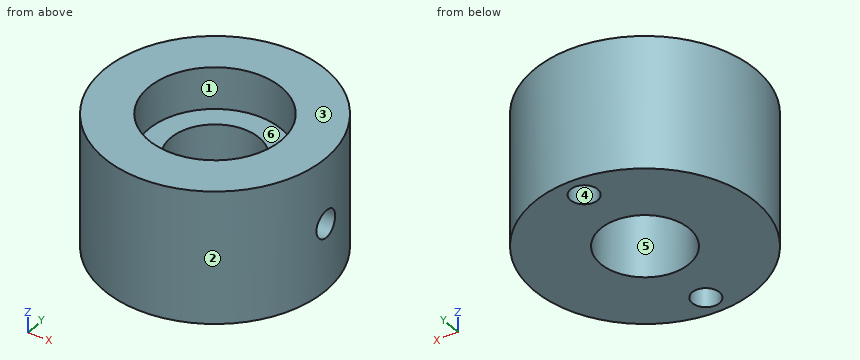
```python
from build123d import *

# Parameters (mm, degrees)
SKETCH1_R               = 15.875
SKETCH1_R_2             = 9.5
BOSS_EXTRUDE1_DEPTH     = 6
BOSS_EXTRUDE2_START     = -13.050000062
SKETCH1_3_R             = 15.875
SKETCH1_3_R_2           = 9.5
SKETCH1_3_R_3           = 6.35
BOSS_EXTRUDE2_DEPTH     = 13.050000062
SKETCH3_R               = 1.95
CUT_EXTRUDE1_DEPTH      = 10.16
CUT_EXTRUDE2_REACH      = 39.82
CUT_EXTRUDE2_END_RADIUS = 9.5


with BuildPart() as part:
    # Sketch1 → Boss-Extrude1 (new body)
    with BuildSketch(Plane.XY):
        Circle(SKETCH1_R)
        Circle(SKETCH1_R_2, mode=Mode.SUBTRACT)
    extrude(amount=BOSS_EXTRUDE1_DEPTH)

    # Sketch1<3> → Boss-Extrude2 (add)
    # profile 1 of 2: a face of its own
    with BuildSketch(Plane.XY.offset(BOSS_EXTRUDE2_START)):
        Circle(SKETCH1_3_R)
        Circle(SKETCH1_3_R_2, mode=Mode.SUBTRACT)
    # profile 2 of 2: a face of its own
    with BuildSketch(Plane.XY.offset(BOSS_EXTRUDE2_START)):
        Circle(SKETCH1_3_R_2)
        Circle(SKETCH1_3_R_3, mode=Mode.SUBTRACT)
    extrude(amount=BOSS_EXTRUDE2_DEPTH)

    # Sketch3 → Cut-Extrude1 (cut)
    with BuildSketch(Plane(origin=(0, 0, -13.050000062), x_dir=(-1, 0, 0), z_dir=(0, 0, -1))):
        with Locations((0, 12.7)):
            Circle(SKETCH3_R)
        with Locations((0, -12.7)):
            Circle(SKETCH3_R)
    extrude(amount=-CUT_EXTRUDE1_DEPTH, mode=Mode.SUBTRACT)

    # Cut-Extrude2: up to this cylinder (the profile starts outside it)
    cut_extrude2_end = Plane(origin=(0, 0, -3.525), z_dir=(0, 0, -1)) * Cylinder(CUT_EXTRUDE2_END_RADIUS, 99.64, mode=Mode.PRIVATE)
    # Sketch4 → Cut-Extrude2 (cut, up to the surface)
    with BuildSketch(Plane(origin=(15.875, 0, 0), x_dir=(0, 0, -1), z_dir=(1, 0, 0)), mode=Mode.PRIVATE) as cut_extrude2_sk1:
        with BuildLine():
            ThreePointArc((5.475000031, 0), (3.525000031, 1.95), (1.575000031, 0))
            Line((1.575000031, 0), (5.475000031, 0))
        make_face()
    cut_extrude2_tool1 = extrude(cut_extrude2_sk1.sketch, amount=-CUT_EXTRUDE2_REACH, mode=Mode.PRIVATE) - cut_extrude2_end
    add(cut_extrude2_tool1.solids().sort_by_distance((15.875, 0.827606, -3.525))[0], mode=Mode.SUBTRACT)
    # Sketch4 → Cut-Extrude2 (cut, up to the surface)
    with BuildSketch(Plane(origin=(15.875, 0, 0), x_dir=(0, 0, -1), z_dir=(1, 0, 0)), mode=Mode.PRIVATE) as cut_extrude2_sk2:
        with BuildLine():
            Line((5.475000031, 0), (1.575000031, 0))
            ThreePointArc((1.575000031, 0), (3.525000031, -1.95), (5.475000031, 0))
        make_face()
    cut_extrude2_tool2 = extrude(cut_extrude2_sk2.sketch, amount=-CUT_EXTRUDE2_REACH, mode=Mode.PRIVATE) - cut_extrude2_end
    add(cut_extrude2_tool2.solids().sort_by_distance((15.875, -0.827606, -3.525))[0], mode=Mode.SUBTRACT)
    # Sketch4 → Cut-Extrude2 (cut, up to the surface)
    with BuildSketch(Plane(origin=(15.875, 0, 0), x_dir=(0, 0, -1), z_dir=(1, 0, 0)), mode=Mode.PRIVATE) as cut_extrude2_sk3:
        with BuildLine():
            ThreePointArc((5.475000031, 0), (3.525000031, 1.95), (1.575000031, 0))
            Line((1.575000031, 0), (5.475000031, 0))
        make_face()
    cut_extrude2_tool3 = extrude(cut_extrude2_sk3.sketch, amount=-CUT_EXTRUDE2_REACH, mode=Mode.PRIVATE) - cut_extrude2_end
    add(cut_extrude2_tool3.solids().sort_by_distance((15.875, 0.827606, -3.525))[0], mode=Mode.SUBTRACT)
    # Sketch4 → Cut-Extrude2 (cut, up to the surface)
    with BuildSketch(Plane(origin=(15.875, 0, 0), x_dir=(0, 0, -1), z_dir=(1, 0, 0)), mode=Mode.PRIVATE) as cut_extrude2_sk4:
        with BuildLine():
            Line((5.475000031, 0), (1.575000031, 0))
            ThreePointArc((1.575000031, 0), (3.525000031, -1.95), (5.475000031, 0))
        make_face()
    cut_extrude2_tool4 = extrude(cut_extrude2_sk4.sketch, amount=-CUT_EXTRUDE2_REACH, mode=Mode.PRIVATE) - cut_extrude2_end
    add(cut_extrude2_tool4.solids().sort_by_distance((15.875, -0.827606, -3.525))[0], mode=Mode.SUBTRACT)


solid = part.part
```
Could you check a few things on this model? Use its own coordinates, in mm. Face numbers are marked on the shaded views. A direction names the side the tool comes from. Give positions to 0.01 mm unless a question says otherwise; leave off trailing zeros. Loops run counter-clockwise (first coordinate to the right, second up) from the corner with the lowest first, then second, coordinate; pieces in that order, holes last. Notation, with made-up numbers: (33, -11.5) - (89, -11.5) arc R22 cw to (89, 12.5) - close; hole circle Ø10 at (81, 43.5). An arc over 180 degrees is marked (long way). Answer in a Markdown table with one row per item. Add a question column.
Q1. For pin 1 (1.2 mm diameter, centred on x = 1, y = -13, fed in from -Z); pin 2 (1.5 mm diameter, centred on y = -7, z = -10, fed in from +X); pin 3 (9.5 mm diameter, centred on x = -3, y = -0.5, fed in from +Z); pin 4 (7.5 mm diameter, centred on x = 0, y = 0, fed in from +Z), each with a flat end and sliding along its axis, tell me the tip position at first contact or that it passes through.
Q2. If we section it at B-B (y = 4): List the corners of the cut face in (x, z) for me.
Q3. Please list where these lines run through material, in increasing order: L1, parallel to Y at x = 0, z = -3 (3 decimals); L2, parallel to Y at x = 0, z = 3.5 (3 decimals); L3, parallel to Y at x = 1, z = -6.75. Write a range as from..to.
Q4. If we section it at D-D (x = 12): List the corners of the cut face in (y, z) for me (3 decimals), plus the area to 3 significant figures.
Q5. If we section it at A-A (x = 0): List the corners of the cut face in (y, z) for me (3 decimals).
Q6. If we section it at C-C (z = -4.5): List the corners of the cut face in (x, y) for me (3 decimals).
Q7. We'd pull the mould along Y, two halves only. Please class the marked faces 1, 2 and 3: +Y half, -Y half, draft (parallel to the pull), parting line (faces both ways), or undercut.
Q8. Which directions (+Z, -Z, +X, -X, +Y, -Y) give clear straight access to the entire face, cutting with the end or side of a thin tool? Please do the marked faces 4, 5 and 6.
The answers:
| question | item | result |
|---|---|---|
| 1 | pin 1 | stops at z = -2.89 |
| 1 | pin 2 | stops at x = 14.59 |
| 1 | pin 3 | stops at z = 0 |
| 1 | pin 4 | passes through |
| 2 | outline | (-15.36, -13.05) - (-4.93, -13.05) - (-4.93, 0) - (-8.62, 0) - (-8.62, 6) - (-15.36, 6) - close; (4.93, -13.05) - (15.36, -13.05) - (15.36, 6) - (8.62, 6) - (8.62, 0) - (4.93, 0) - close |
| 3 | L1 | y = -15.875..-14.65, -10.75..-6.35, 6.35..10.75, 14.65..15.875 |
| 3 | L2 | y = -15.875..-9.5, 9.5..15.875 |
| 3 | L3 | y = -15.84..-14.37, -11.03..-6.27, 6.27..11.03, 14.37..15.84 |
| 4 | outline | (-10.393, -13.05) - (10.393, -13.05) - (10.393, 6) - (-10.393, 6) - close; hole circle Ø3.9 at (0, -3.525) |
| 4 | area | 384 mm^2 |
| 5 | outline | (-15.875, -13.05) - (-14.65, -13.05) - (-14.65, -2.89) - (-10.75, -2.89) - (-10.75, -13.05) - (-6.35, -13.05) - (-6.35, 0) - (-9.5, 0) - (-9.5, 6) - (-15.875, 6) - close; (6.35, -13.05) - (10.75, -13.05) - (10.75, -2.89) - (14.65, -2.89) - (14.65, -13.05) - (15.875, -13.05) - (15.875, 6) - (9.5, 6) - (9.5, 0) - (6.35, 0) - close |
| 6 | outline | (9.349, -1.689) arc R9.5 ccw to (9.349, 1.689) - (15.785, 1.689) arc R15.875 ccw (long way) to (15.785, -1.689) - close; hole circle Ø12.7 at (0, 0); hole circle Ø3.9 at (0, -12.7); hole circle Ø3.9 at (0, 12.7) |
| 7 | face 1 | undercut |
| 7 | face 2 | parting line |
| 7 | face 3 | draft |
| 8 | face 4 | -Z |
| 8 | face 5 | +Z, -Z |
| 8 | face 6 | +Z |
